Read the model definition and answer for the solid it produces. Units are mm, in the model's axes. A direction names the side the tool comes from. Coordinates: 2 decimals unless noted, no trailing zeros. Order: outer loops, then holes, each group sorted by start corner. A loop starts at its lowest first (then second) coordinate and runs counter-clockwise, first axis right, second up. Notation, with made-up numbers: M 24.5,0 L 71.5,0 A30 cw 71.5,29 Z; hole C -10.75,79.25 d5. An arc over 180 degrees is marked long. One line per question, with ' | ' between items. Start each with the question number.
1) Find section C-C, the plane x = 25.4. Write down the section's boundary in (y, z).
2) Consider probe 1 along Y at (x, z) = (0, 12); probe 2 along Y at (x, z) = (25, 24); probe 3 along Z at (x, y) = (-9, 4.5). Determine where each line is inside the solid, lowest interval first.
3) Find section B-B, the plane z = 42. Write down the section's boundary in (x, y), plus the area to 3 significant figures.
4) Given P1, Ø12, axis at y = -22.5, z = 36.5, coming from the +X side; P2, Ø2, axis at x = -23, z = 16.5, coming from the -Y side; P3, Ø4, axis at y = -15, z = 28, coming from the +X side; P4, Ø2.5, axis at x = 0, y = -25.4, coming from the -Z side, each flat-ended and moving along its own axis, determine where each tip first touches the part or whether it passes through.
5) A tool of negligible diameter and unlimited length cuts with its end or side. For faces 4 (the face through (-2.75, -12.4, 38.28)), 5 (the face through (0.267, -23.367, 25.044)), from which of +Z, -Z, +X, -X, +Y, -Y can it reach the whole face along a straight path? Write none if from no direction.
6) Find section A-A, the plane y = 0. Write down the section's boundary in (x, z).
7) The mould has two halves that part along X. Classify faces 1 (the face through (-1, 1, 0)), 2 (the face through (0, 0, 25.4)), 3 (the face through (-30.235, -23.183, 25.044)): +X half, -X half, draft (parallel to the pull), parting line (faces both ways), or undercut.
from build123d import *

# Parameters (mm, degrees)
F0_R     = 38.1
F1_DEPTH = 50.8
F2_R     = 12.7
F3_DEPTH = 25.4
F5_D     = 4.1


with BuildPart() as f1:
    # F0 (on Top) → F1 (new body)
    with BuildSketch(Plane.XY):
        Circle(F0_R)
    extrude(amount=F1_DEPTH)

    # F2 (on face) → F3 (cut)
    with BuildSketch(Plane.XY.offset(50.8)):
        Circle(F2_R)
    extrude(amount=-F3_DEPTH, mode=Mode.SUBTRACT)

    # F5 (through all)
    with Locations(Plane.XY.offset(50.8)):
        with Locations((25.4, 0), (0, 25.4), (-25.4, 0), (0, -25.4)):
            Hole(F5_D / 2)


solid = f1.part
Report:
1) outline: M -28.4,0 L -2.05,0 L -2.05,50.8 L -28.4,50.8 Z; M 2.05,0 L 28.4,0 L 28.4,50.8 L 2.05,50.8 Z
2) probe 1: y = -38.1 to -27.45, -23.35 to 23.35, 27.45 to 38.1 | probe 2: y = -28.75 to -2.01, 2.01 to 28.75 | probe 3: z = 0 to 25.4
3) outline: C 0,0 d76.2; hole C -25.4,0 d4.1; hole C 0,0 d25.4; hole C 0,-25.4 d4.1; hole C 0,25.4 d4.1; hole C 25.4,0 d4.1 | area: 4,000 mm^2
4) P1: stops at x = 34.34 | P2: stops at y = -31.11 | P3: stops at x = 35.81 | P4: passes through
5) face 4: +Z | face 5: +Z, -Z
6) outline: M -38.1,0 L -27.45,0 L -27.45,50.8 L -38.1,50.8 Z; M -23.35,0 L 23.35,0 L 23.35,50.8 L 12.7,50.8 L 12.7,25.4 L -12.7,25.4 L -12.7,50.8 L -23.35,50.8 Z; M 27.45,0 L 38.1,0 L 38.1,50.8 L 27.45,50.8 Z
7) face 1: draft | face 2: undercut | face 3: parting line
